Work out the finished part from the listing and answer in its coordinate system (mm). Face numbers are marked on the shaded views. Coordinates: 2 decimals unless noted, no trailing zeros. Order: outer loops, then holes, each group sorted by start corner. A loop starts at its lowest first (then second) coordinate and runs counter-clockwise, first axis right, second up. Notation, with made-up numbers: M 51.5,19.25 L 89.5,19.25 A30 cw 89.5,57.25 Z; hole C 77.25,-1.5 d6. An arc over 180 degrees is marked long. Answer in a Markdown table with one row per item. Add a question column.
Item 1: The part is cut by section A-A (x = -31). Write down the section's boundary in (y, z).
Item 2: Consider line 1 (X direction, y = 92, z = 26.4); line 2 (Z direction, x = 0.5, y = 88); line 3 (Y direction, x = -31, z = 22.75). Determine where each line is inside the solid, lowest interval first. Write a range as from..to.
Item 3: The part is cut by section B-B (x = 0). Write down the section's boundary in (y, z).
Item 4: The part is cut by section D-D (y = 113). Write down the section's boundary in (x, z), then the cut area to 3 significant figures.
Item 5: The part is cut by section C-C (z = 25.7). Write down the section's boundary in (x, y), then the cut area to 3 significant figures.
Item 6: Flat-ended cylindrical pins translate along their axes: pin 1 Ø1.7 at (x, y) = (30, 91.5) entering from -Z; pin 2 Ø1 at (x, z) = (23, 26) entering from +Y; pin 3 Ø4.5 at (x, y) = (-32, 93.5) entering from -Z; pin 4 Ø2 at (y, z) = (103, 25) entering from +X. Find the tip coordinate at first contact, or state that the pin passes through.
Item 7: The mould has two halves that part along X. Classify the marked faces 1, 2 and 3: released by +X, released by -X, zero draft, split by the parting line, or undercut.
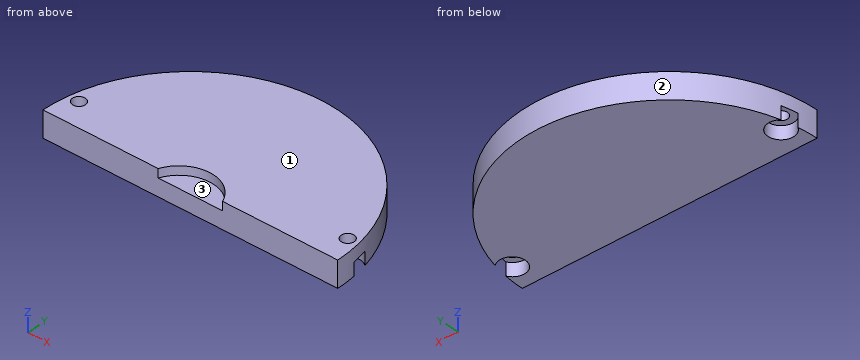
from build123d import *

# Parameters (mm, degrees)
CYLINDER687_R               = 8
CYLINDER687_DEPTH           = 6
CYLINDER688_R               = 3
CYLINDER688_DEPTH           = 3
CYLINDER688_PLACEMENT_ANGLE = 45
CYLINDER668_R               = 3
CYLINDER668_DEPTH           = 3
CYLINDER668_PLACEMENT_ANGLE = 45
CYLINDER676_R               = 3
CYLINDER676_DEPTH           = 3
CYLINDER676_PLACEMENT_ANGLE = 45
CYLINDER683_R               = 3
CYLINDER683_DEPTH           = 3
CYLINDER683_PLACEMENT_ANGLE = 45
CYLINDER681_R               = 1.5
CYLINDER681_DEPTH           = 50
CYLINDER681_PLACEMENT_ANGLE = 45
CYLINDER686_R               = 1.5
CYLINDER686_DEPTH           = 50
CYLINDER686_PLACEMENT_ANGLE = 45
CYLINDER685_R               = 1.5
CYLINDER685_DEPTH           = 50
CYLINDER685_PLACEMENT_ANGLE = 45
CYLINDER675_R               = 1.5
CYLINDER675_DEPTH           = 50
CYLINDER675_PLACEMENT_ANGLE = 45
BOX250_W                    = 148
BOX250_H                    = 40
BOX250_DEPTH                = 40
CYLINDER671_R               = 34
CYLINDER671_DEPTH           = 6


with BuildPart() as obj1:
    # Cylinder687 → Cylinder687 (new body)
    with BuildSketch(Plane(origin=(0, 83, 25), x_dir=(1, 0, 0), z_dir=(0, 0, 1))):
        Circle(CYLINDER687_R)
    extrude(amount=CYLINDER687_DEPTH)


with BuildPart() as obj2:
    # Cylinder688 → Cylinder688 (new body)
    with BuildSketch(Plane.XY):
        Circle(CYLINDER688_R)
    extrude(amount=CYLINDER688_DEPTH)


with BuildPart() as obj2_1:
    # Cylinder688 placement: moved
    add(obj2.part.moved(Location((-31, 92, 21))).rotate(Axis((-31, 92, 21), (0, 0, 1)), CYLINDER688_PLACEMENT_ANGLE))


with BuildPart() as obj3:
    # Cylinder668 → Cylinder668 (new body)
    with BuildSketch(Plane.XY):
        Circle(CYLINDER668_R)
    extrude(amount=CYLINDER668_DEPTH)


with BuildPart() as obj3_1:
    # Cylinder668 placement: moved
    add(obj3.part.moved(Location((31, 110, 0))).rotate(Axis((31, 110, 0), (0, 0, 1)), CYLINDER668_PLACEMENT_ANGLE))


with BuildPart() as obj4:
    # Cylinder676 → Cylinder676 (new body)
    with BuildSketch(Plane.XY):
        Circle(CYLINDER676_R)
    extrude(amount=CYLINDER676_DEPTH)


with BuildPart() as obj4_1:
    # Cylinder676 placement: moved
    add(obj4.part.moved(Location((31, 92, 21))).rotate(Axis((31, 92, 21), (0, 0, 1)), CYLINDER676_PLACEMENT_ANGLE))


with BuildPart() as compound400:
    # Cylinder683 → Cylinder683 (new body)
    with BuildSketch(Plane.XY):
        Circle(CYLINDER683_R)
    extrude(amount=CYLINDER683_DEPTH)


with BuildPart() as compound400_1:
    # Cylinder683 placement: moved
    add(compound400.part.moved(Location((-31, 110, 0))).rotate(Axis((-31, 110, 0), (0, 0, 1)), CYLINDER683_PLACEMENT_ANGLE))

    # Compound400: union obj2, obj3, obj4
    add(obj2_1.part)
    add(obj3_1.part)
    add(obj4_1.part)


with BuildPart() as obj5:
    # Cylinder681 → Cylinder681 (new body)
    with BuildSketch(Plane.XY):
        Circle(CYLINDER681_R)
    extrude(amount=CYLINDER681_DEPTH)


with BuildPart() as obj5_1:
    # Cylinder681 placement: moved
    add(obj5.part.moved(Location((-31, 92, 0))).rotate(Axis((-31, 92, 0), (0, 0, 1)), CYLINDER681_PLACEMENT_ANGLE))


with BuildPart() as obj6:
    # Cylinder686 → Cylinder686 (new body)
    with BuildSketch(Plane.XY):
        Circle(CYLINDER686_R)
    extrude(amount=CYLINDER686_DEPTH)


with BuildPart() as obj6_1:
    # Cylinder686 placement: moved
    add(obj6.part.moved(Location((31, 110, 0))).rotate(Axis((31, 110, 0), (0, 0, 1)), CYLINDER686_PLACEMENT_ANGLE))


with BuildPart() as obj7:
    # Cylinder685 → Cylinder685 (new body)
    with BuildSketch(Plane.XY):
        Circle(CYLINDER685_R)
    extrude(amount=CYLINDER685_DEPTH)


with BuildPart() as obj7_1:
    # Cylinder685 placement: moved
    add(obj7.part.moved(Location((31, 92, 0))).rotate(Axis((31, 92, 0), (0, 0, 1)), CYLINDER685_PLACEMENT_ANGLE))


with BuildPart() as compound396:
    # Cylinder675 → Cylinder675 (new body)
    with BuildSketch(Plane.XY):
        Circle(CYLINDER675_R)
    extrude(amount=CYLINDER675_DEPTH)


with BuildPart() as compound396_1:
    # Cylinder675 placement: moved
    add(compound396.part.moved(Location((-31, 110, 0))).rotate(Axis((-31, 110, 0), (0, 0, 1)), CYLINDER675_PLACEMENT_ANGLE))

    # Compound396: union obj5, obj6, obj7
    add(obj5_1.part)
    add(obj6_1.part)
    add(obj7_1.part)


with BuildPart() as krychle250:
    # Box250 → Box250 (new body)
    with BuildSketch(Plane(origin=(-74, 46, 16), x_dir=(1, 0, 0), z_dir=(0, 0, 1))):
        with Locations((74, 20)):
            Rectangle(BOX250_W, BOX250_H)
    extrude(amount=BOX250_DEPTH)


with BuildPart() as cut274:
    # Cylinder671 → Cylinder671 (new body)
    with BuildSketch(Plane(origin=(0, 86, 21), x_dir=(1, 0, 0), z_dir=(0, 0, 1))):
        Circle(CYLINDER671_R)
    extrude(amount=CYLINDER671_DEPTH)

    # Cut271: cut Krychle250
    add(krychle250.part, mode=Mode.SUBTRACT)

    # Cut277: cut Compound396
    add(compound396_1.part, mode=Mode.SUBTRACT)

    # Cut275: cut Compound400
    add(compound400_1.part, mode=Mode.SUBTRACT)

    # Cut274: cut obj1
    add(obj1.part, mode=Mode.SUBTRACT)


solid = cut274.part
Reply:
| question | item | result |
|---|---|---|
| 1 | outline | M 86,21 L 89,21 L 89,24 L 90.5,24 L 90.5,27 L 86,27 Z; M 93.5,24 L 95,24 L 95,21 L 99.96,21 L 99.96,27 L 93.5,27 Z |
| 2 | line 1 | x = -33.47..-32.5, -29.5..29.5, 32.5..33.47 |
| 2 | line 2 | z = 21..25 |
| 2 | line 3 | y = 86..89, 95..99.96 |
| 3 | outline | M 86,21 L 120,21 L 120,27 L 91,27 L 91,25 L 86,25 Z |
| 4 | outline | M -20.66,21 L 20.66,21 L 20.66,27 L -20.66,27 Z |
| 4 | area | 248 mm2 |
| 5 | outline | M -34,86 L -7.42,86 A8 cw 7.42,86 L 34,86 A34 ccw Z; hole C -31,92 d3; hole C 31,92 d3 |
| 5 | area | 1,750 mm2 |
| 6 | pin 1 | stops at z = 24 |
| 6 | pin 2 | stops at y = 111.49 |
| 6 | pin 3 | stops at z = 21 |
| 6 | pin 4 | stops at x = 30 |
| 7 | face 1 | zero draft |
| 7 | face 2 | split by the parting line |
| 7 | face 3 | undercut |
